For this review, take the finished solid that the model builds, in its own axes (mm). A direction names the side the tool comes from. Coordinates: 2 decimals unless noted, no trailing zeros. Write each loop counter-clockwise with the first axis right and the second up, starting at its lowest first coordinate (ties: lowest second). Pieces come first, ordered by that corner, then holes.
```python
from build123d import *

# Parameters (mm, degrees)
SKETCH_0_R   = 7.5
PAD_DEPTH    = 10
SKETCH_2_W   = 200
SKETCH_2_H   = 20
PAD001_DEPTH = 85
SKETCH_1_R   = 7.5
PAD002_DEPTH = 10


with BuildPart() as part:
    with BuildSketch(Plane.YZ):
        with BuildLine():
            ThreePointArc((23.973718, 7.089487), (0, 25), (-23.973718, 7.089487))
            Line((-23.973718, 7.089487), (-100, -250))
            Line((-100, -250), (100, -250))
            Line((23.973718, 7.089487), (100, -250))
        make_face()
        Circle(SKETCH_0_R, mode=Mode.SUBTRACT)
    extrude(amount=PAD_DEPTH)

    with BuildSketch(Plane.YZ):
        with Locations((0, -260)):
            Rectangle(SKETCH_2_W, SKETCH_2_H)
    extrude(amount=PAD001_DEPTH)

    with BuildSketch(Plane(origin=(85, 0, -100), x_dir=(0, 1, 0), z_dir=(1, 0, 0))):
        with BuildLine():
            ThreePointArc((20, -15), (0, 25), (-20, -15))
            Line((-100, -150), (-20, -15))
            Line((100, -150), (-100, -150))
            Line((20, -15), (100, -150))
        make_face()
        Circle(SKETCH_1_R, mode=Mode.SUBTRACT)
    extrude(amount=-PAD002_DEPTH)


solid = part.part
```
Q1. Add section A-A (y = 0). State the section outline as (x, z) points, then the cut area to 3 significant figures.
Ans:
outline: (0, -270) - (85, -270) - (85, -107.5) - (75, -107.5) - (75, -250) - (10, -250) - (10, -7.5) - (0, -7.5) - close; (0, 7.5) - (10, 7.5) - (10, 25) - (0, 25) - close; (75, -92.5) - (85, -92.5) - (85, -75) - (75, -75) - close
area: 5,900 mm2
Q2. Add section C-C (x = 79). State the section outline as (y, z) points.
Ans:
outline: (-100, -270) - (100, -270) - (100, -250) - (20, -115) arc R25 ccw (long way) to (-20, -115) - (-100, -250) - close; hole circle Ø15 at (0, -100)
Q3. For probe 1 along X at (y, z) = (-50, -235.5); probe 2 along X at (y, z) = (27, -55.5); probe 3 along Z at (x, y) = (71, -50), list the stretches that pass through material, from the lowest coordinate up.
Ans:
probe 1: x = 0 to 10, 75 to 85
probe 2: x = 0 to 10
probe 3: z = -270 to -250
Q4. Draft analysis for pull direction Z (two halves, no side actions). For faces 1 (the cylindrical face through (80.07, -1.63, -107.32)), 2 (the flat face through (42, -1, -270)), 3 (the cylindrical face through (4.93, -7.493, 0.33)), 4 (the flat face through (85, -1, -193)), state which applies: +Z half, -Z half, draft (parallel to the pull), parting line (faces both ways), or undercut.
Ans:
face 1: undercut
face 2: -Z half
face 3: undercut
face 4: draft
Q5. Add section D-D (z = 0). State the section outline as (x, y) points.
Ans:
outline: (0, -26.07) - (10, -26.07) - (10, -7.5) - (0, -7.5) - close; (0, 7.5) - (10, 7.5) - (10, 26.07) - (0, 26.07) - close
Q6. Tool access review of faces 5 (the cylindrical face through (5, 0, 25)), 6 (the cylindrical face through (80.07, 0.77, -75.01)), 7 (the flat face through (42, -1, -250)): name each direction out of +Z, -Z, +X, -X, +Y, -Y from which nothing blocks a thin tool from reaching the whole face with its end or side.
Ans:
face 5: +Z, +X, -X
face 6: +X
face 7: +Z, +Y, -Y
Q7. Add section B-B (z = -100). State the section outline as (x, y) points.
Ans:
outline: (0, -55.64) - (10, -55.64) - (10, 55.64) - (0, 55.64) - close; (75, -25) - (85, -25) - (85, -7.5) - (75, -7.5) - close; (75, 7.5) - (85, 7.5) - (85, 25) - (75, 25) - close
Q8. Clearance check with a flat-ended pin moving along its axis: pin 1 Ø1.5 at (y, z) = (-56.5, -142) entering from +X. State where the tip first meets the part, or that it passes through.
Ans:
pin 1: stops at x = 10
